Check sheet for the modelled part. Datum: model origin and axes. Units: mm. A direction names the side the tool comes from. Give positions to 0.01 mm unless a question says otherwise; leave off trailing zeros. Write each loop counter-clockwise with the first axis right and the second up, starting at its lowest first coordinate (ties: lowest second). Pieces come first, ordered by that corner, then holes. Notation, with made-up numbers: (-24, 56.5) -> (6, 56.5) arc R10 ccw to (6, 64.5) -> close; hole circle Ø9 at (63.25, 27.25). An arc over 180 degrees is marked (long way). Answer as a JSON object with one key per item and string values.
from build123d import *

# Parameters (mm, degrees)
F1_DEPTH = 41


with BuildPart() as f1:
    # F0 (on Front) → F1 (new body)
    with BuildSketch(Plane.XZ):
        Polygon((1, 6), (0, 6), (0, 0), (41, 0), (41, 6), (40, 6), (40, 5), (39, 5), (39, 6), (38.5, 6), (38.5, 5), (37.5, 5), (37.5, 6), (37, 6), (37, 5), (36, 5), (36, 6), (35, 6), (35, 5), (34, 5), (34, 6), (33.5, 6), (33.5, 5), (32.5, 5), (32.5, 6), (32, 6), (32, 5), (31, 5), (31, 6), (30, 6), (30, 5), (29, 5), (29, 6), (28.5, 6), (28.5, 5), (27.5, 5), (27.5, 6), (27, 6), (27, 5), (26, 5), (26, 6), (25, 6), (25, 5), (24, 5), (24, 6), (23.5, 6), (23.5, 5), (22.5, 5), (22.5, 6), (22, 6), (22, 5), (21, 5), (21, 6), (20, 6), (20, 5), (19, 5), (19, 6), (18.5, 6), (18.5, 5), (17.5, 5), (17.5, 6), (17, 6), (17, 5), (16, 5), (16, 6), (15, 6), (15, 5), (14, 5), (14, 6), (13.5, 6), (13.5, 5), (12.5, 5), (12.5, 6), (12, 6), (12, 5), (11, 5), (11, 6), (10, 6), (10, 5), (9, 5), (9, 6), (8.5, 6), (8.5, 5), (7.5, 5), (7.5, 6), (7, 6), (7, 5), (6, 5), (6, 6), (5, 6), (5, 5), (4, 5), (4, 6), (3.5, 6), (3.5, 5), (2.5, 5), (2.5, 6), (2, 6), (2, 5), (1, 5), align=None)
    extrude(amount=F1_DEPTH)


solid = f1.part
1. Go/stop test with a flat-tipped pin: P1, Ø0.8, axis at x = 34.5, y = -19, coming from the +Z side. Record where the tip stops, or that it passes through.
Determined:
{"P1": "z = 5"}
2. Access from +Z, -Z, +X, -X, +Y, -Y to the whole of each face (thin tool, end or side, straight path). Record for faces 1 (the face through (5.5, -20.2, 6)), 2 (the face through (6.5, -20.2, 5)).
Determined:
{"face 1": "+Z, +X, -X, +Y, -Y", "face 2": "+Z, +Y, -Y"}
3. Scan line: L1, parallel to Z at x = 8, y = -14. Record every from-to range of solid material in increasing order. Write a range as [from, to].
Determined:
{"L1": "[0, 5]"}
4. Mould release check, pull along X, two halves, no side actions. Record for faces 3 (the face through (15.5, -20.2, 6)), 4 (the face through (0, -20, 3)), 5 (the face through (16.5, -20.2, 5)): released by +X, released by -X, zero draft, split by the parting line, or undercut.
Determined:
{"face 3": "zero draft", "face 4": "released by -X", "face 5": "undercut"}
5. Sectioned sample at A-A, the plane x = 34.5. Enter the section's corners in (y, z).
Determined:
{"outline": "(-41, 0) -> (0, 0) -> (0, 5) -> (-41, 5) -> close"}
